Design review of the part built by this model. Coordinates are the model's own, in mm. Coordinates: 2 decimals unless noted, no trailing zeros. Order: outer loops, then holes, each group sorted by start corner. A loop starts at its lowest first (then second) coordinate and runs counter-clockwise, first axis right, second up. Notation, with made-up numbers: M 3.5,60.25 L 36.5,60.25 A26 ccw 36.5,79.25 Z; hole C 69.5,65.25 d4. An arc over 180 degrees is marked long. Answer in a Markdown table with one row per item.
from build123d import *

# Parameters (mm, degrees)
F1_DEPTH = 6.35


with BuildPart() as f1:
    # F0 (on Front) → F1 (new body)
    with BuildSketch(Plane.XZ):
        Polygon((-100.167322, -14.499216), (-100.167322, 36.300784), (-94.868163, 36.300784), (-88.733239, 36.300784), (-82.168163, 36.300784), (-76.033239, 36.300784), (-69.468163, 36.300784), (-63.333239, 36.300784), (-56.768163, 36.300784), (-50.633239, 36.300784), (-44.068163, 36.300784), (-37.933239, 36.300784), (-31.368163, 36.300784), (-25.233239, 36.300784), (-18.668163, 36.300784), (-12.533239, 36.300784), (-5.968163, 36.300784), (0.166761, 36.300784), (6.731837, 36.300784), (12.866761, 36.300784), (19.431837, 36.300784), (25.566761, 36.300784), (32.131837, 36.300784), (38.266761, 36.300784), (44.831837, 36.300784), (50.966761, 36.300784), (57.531837, 36.300784), (63.666761, 36.300784), (70.231837, 36.300784), (76.366761, 36.300784), (82.931837, 36.300784), (89.066761, 36.300784), (95.631837, 36.300784), (101.766761, 36.300784), (103.032678, 36.300784), (103.032678, 39.458872), (-106.993854, 39.458872), (-106.993854, -18.961128), (103.032678, -18.961128), (103.032678, -14.499216), (101.766761, -14.499216), (95.631837, -14.499216), (89.066761, -14.499216), (82.931837, -14.499216), (76.366761, -14.499216), (70.231837, -14.499216), (63.666761, -14.499216), (57.531837, -14.499216), (50.966761, -14.499216), (44.831837, -14.499216), (38.266761, -14.499216), (32.131837, -14.499216), (25.566761, -14.499216), (19.431837, -14.499216), (12.866761, -14.499216), (6.731837, -14.499216), (0.166761, -14.499216), (-5.968163, -14.499216), (-12.533239, -14.499216), (-18.668163, -14.499216), (-25.233239, -14.499216), (-31.368163, -14.499216), (-37.933239, -14.499216), (-44.068163, -14.499216), (-50.633239, -14.499216), (-56.768163, -14.499216), (-63.333239, -14.499216), (-69.468163, -14.499216), (-76.033239, -14.499216), (-82.168163, -14.499216), (-88.733239, -14.499216), (-94.868163, -14.499216), align=None)
        with BuildLine():
            Line((-88.733239, 36.300784), (-94.868163, 36.300784))
            ThreePointArc((-94.868163, 36.300784), (-94.016162, 33.181807), (-91.696805, 30.92914))
            ThreePointArc((-91.696805, 30.92914), (-89.523277, 33.233322), (-88.733239, 36.300784))
        make_face()
        with BuildLine():
            Line((-76.033239, 36.300784), (-82.168163, 36.300784))
            ThreePointArc((-82.168163, 36.300784), (-81.316162, 33.181807), (-78.996805, 30.92914))
            ThreePointArc((-78.996805, 30.92914), (-76.823277, 33.233322), (-76.033239, 36.300784))
        make_face()
        with BuildLine():
            Line((-63.333239, 36.300784), (-69.468163, 36.300784))
            ThreePointArc((-69.468163, 36.300784), (-68.616162, 33.181807), (-66.296805, 30.92914))
            ThreePointArc((-66.296805, 30.92914), (-64.123277, 33.233322), (-63.333239, 36.300784))
        make_face()
        with BuildLine():
            Line((-50.633239, 36.300784), (-56.768163, 36.300784))
            ThreePointArc((-56.768163, 36.300784), (-55.916162, 33.181807), (-53.596805, 30.92914))
            ThreePointArc((-53.596805, 30.92914), (-51.423277, 33.233322), (-50.633239, 36.300784))
        make_face()
        with BuildLine():
            Line((-37.933239, 36.300784), (-44.068163, 36.300784))
            ThreePointArc((-44.068163, 36.300784), (-43.216162, 33.181807), (-40.896805, 30.92914))
            ThreePointArc((-40.896805, 30.92914), (-38.723277, 33.233322), (-37.933239, 36.300784))
        make_face()
        with BuildLine():
            Line((-25.233239, 36.300784), (-31.368163, 36.300784))
            ThreePointArc((-31.368163, 36.300784), (-30.516162, 33.181807), (-28.196805, 30.92914))
            ThreePointArc((-28.196805, 30.92914), (-26.023277, 33.233322), (-25.233239, 36.300784))
        make_face()
        with BuildLine():
            Line((-12.533239, 36.300784), (-18.668163, 36.300784))
            ThreePointArc((-18.668163, 36.300784), (-17.816162, 33.181807), (-15.496805, 30.92914))
            ThreePointArc((-15.496805, 30.92914), (-13.323277, 33.233322), (-12.533239, 36.300784))
        make_face()
        with BuildLine():
            Line((0.166761, 36.300784), (-5.968163, 36.300784))
            ThreePointArc((-5.968163, 36.300784), (-5.116162, 33.181807), (-2.796805, 30.92914))
            ThreePointArc((-2.796805, 30.92914), (-0.623277, 33.233322), (0.166761, 36.300784))
        make_face()
        with BuildLine():
            Line((12.866761, 36.300784), (6.731837, 36.300784))
            ThreePointArc((6.731837, 36.300784), (7.583838, 33.181807), (9.903195, 30.92914))
            ThreePointArc((9.903195, 30.92914), (12.076723, 33.233322), (12.866761, 36.300784))
        make_face()
        with BuildLine():
            Line((25.566761, 36.300784), (19.431837, 36.300784))
            ThreePointArc((19.431837, 36.300784), (20.283838, 33.181807), (22.603195, 30.92914))
            ThreePointArc((22.603195, 30.92914), (24.776723, 33.233322), (25.566761, 36.300784))
        make_face()
        with BuildLine():
            Line((38.266761, 36.300784), (32.131837, 36.300784))
            ThreePointArc((32.131837, 36.300784), (32.983838, 33.181807), (35.303195, 30.92914))
            ThreePointArc((35.303195, 30.92914), (37.476723, 33.233322), (38.266761, 36.300784))
        make_face()
        with BuildLine():
            Line((50.966761, 36.300784), (44.831837, 36.300784))
            ThreePointArc((44.831837, 36.300784), (45.683838, 33.181807), (48.003195, 30.92914))
            ThreePointArc((48.003195, 30.92914), (50.176723, 33.233322), (50.966761, 36.300784))
        make_face()
        with BuildLine():
            Line((63.666761, 36.300784), (57.531837, 36.300784))
            ThreePointArc((57.531837, 36.300784), (58.383838, 33.181807), (60.703195, 30.92914))
            ThreePointArc((60.703195, 30.92914), (62.876723, 33.233322), (63.666761, 36.300784))
        make_face()
        with BuildLine():
            Line((76.366761, 36.300784), (70.231837, 36.300784))
            ThreePointArc((70.231837, 36.300784), (71.083838, 33.181807), (73.403195, 30.92914))
            ThreePointArc((73.403195, 30.92914), (75.576723, 33.233322), (76.366761, 36.300784))
        make_face()
        with BuildLine():
            Line((89.066761, 36.300784), (82.931837, 36.300784))
            ThreePointArc((82.931837, 36.300784), (83.783838, 33.181807), (86.103195, 30.92914))
            ThreePointArc((86.103195, 30.92914), (88.276723, 33.233322), (89.066761, 36.300784))
        make_face()
        with BuildLine():
            Line((101.766761, 36.300784), (95.631837, 36.300784))
            ThreePointArc((95.631837, 36.300784), (96.483838, 33.181807), (98.803195, 30.92914))
            ThreePointArc((98.803195, 30.92914), (100.976723, 33.233322), (101.766761, 36.300784))
        make_face()
        with BuildLine():
            ThreePointArc((98.803195, -9.127571), (96.483838, -11.380239), (95.631837, -14.499216))
            Line((95.631837, -14.499216), (101.766761, -14.499216))
            ThreePointArc((101.766761, -14.499216), (100.976723, -11.431754), (98.803195, -9.127571))
        make_face()
        with BuildLine():
            ThreePointArc((86.103195, -9.127571), (83.783838, -11.380239), (82.931837, -14.499216))
            Line((82.931837, -14.499216), (89.066761, -14.499216))
            ThreePointArc((89.066761, -14.499216), (88.276723, -11.431754), (86.103195, -9.127571))
        make_face()
        with BuildLine():
            ThreePointArc((73.403195, -9.127571), (71.083838, -11.380239), (70.231837, -14.499216))
            Line((70.231837, -14.499216), (76.366761, -14.499216))
            ThreePointArc((76.366761, -14.499216), (75.576723, -11.431754), (73.403195, -9.127571))
        make_face()
        with BuildLine():
            ThreePointArc((60.703195, -9.127571), (58.383838, -11.380239), (57.531837, -14.499216))
            Line((57.531837, -14.499216), (63.666761, -14.499216))
            ThreePointArc((63.666761, -14.499216), (62.876723, -11.431754), (60.703195, -9.127571))
        make_face()
        with BuildLine():
            ThreePointArc((48.003195, -9.127571), (45.683838, -11.380239), (44.831837, -14.499216))
            Line((44.831837, -14.499216), (50.966761, -14.499216))
            ThreePointArc((50.966761, -14.499216), (50.176723, -11.431754), (48.003195, -9.127571))
        make_face()
        with BuildLine():
            ThreePointArc((35.303195, -9.127571), (32.983838, -11.380239), (32.131837, -14.499216))
            Line((32.131837, -14.499216), (38.266761, -14.499216))
            ThreePointArc((38.266761, -14.499216), (37.476723, -11.431754), (35.303195, -9.127571))
        make_face()
        with BuildLine():
            ThreePointArc((22.603195, -9.127571), (20.283838, -11.380239), (19.431837, -14.499216))
            Line((19.431837, -14.499216), (25.566761, -14.499216))
            ThreePointArc((25.566761, -14.499216), (24.776723, -11.431754), (22.603195, -9.127571))
        make_face()
        with BuildLine():
            ThreePointArc((9.903195, -9.127571), (7.583838, -11.380239), (6.731837, -14.499216))
            Line((6.731837, -14.499216), (12.866761, -14.499216))
            ThreePointArc((12.866761, -14.499216), (12.076723, -11.431754), (9.903195, -9.127571))
        make_face()
        with BuildLine():
            ThreePointArc((-2.796805, -9.127571), (-5.116162, -11.380239), (-5.968163, -14.499216))
            Line((-5.968163, -14.499216), (0.166761, -14.499216))
            ThreePointArc((0.166761, -14.499216), (-0.623277, -11.431754), (-2.796805, -9.127571))
        make_face()
        with BuildLine():
            ThreePointArc((-15.496805, -9.127571), (-17.816162, -11.380239), (-18.668163, -14.499216))
            Line((-18.668163, -14.499216), (-12.533239, -14.499216))
            ThreePointArc((-12.533239, -14.499216), (-13.323277, -11.431754), (-15.496805, -9.127571))
        make_face()
        with BuildLine():
            ThreePointArc((-28.196805, -9.127571), (-30.516162, -11.380239), (-31.368163, -14.499216))
            Line((-31.368163, -14.499216), (-25.233239, -14.499216))
            ThreePointArc((-25.233239, -14.499216), (-26.023277, -11.431754), (-28.196805, -9.127571))
        make_face()
        with BuildLine():
            ThreePointArc((-40.896805, -9.127571), (-43.216162, -11.380239), (-44.068163, -14.499216))
            Line((-44.068163, -14.499216), (-37.933239, -14.499216))
            ThreePointArc((-37.933239, -14.499216), (-38.723277, -11.431754), (-40.896805, -9.127571))
        make_face()
        with BuildLine():
            ThreePointArc((-53.596805, -9.127571), (-55.916162, -11.380239), (-56.768163, -14.499216))
            Line((-56.768163, -14.499216), (-50.633239, -14.499216))
            ThreePointArc((-50.633239, -14.499216), (-51.423277, -11.431754), (-53.596805, -9.127571))
        make_face()
        with BuildLine():
            ThreePointArc((-66.296805, -9.127571), (-68.616162, -11.380239), (-69.468163, -14.499216))
            Line((-69.468163, -14.499216), (-63.333239, -14.499216))
            ThreePointArc((-63.333239, -14.499216), (-64.123277, -11.431754), (-66.296805, -9.127571))
        make_face()
        with BuildLine():
            ThreePointArc((-78.996805, -9.127571), (-81.316162, -11.380239), (-82.168163, -14.499216))
            Line((-82.168163, -14.499216), (-76.033239, -14.499216))
            ThreePointArc((-76.033239, -14.499216), (-76.823277, -11.431754), (-78.996805, -9.127571))
        make_face()
        with BuildLine():
            ThreePointArc((-91.696805, -9.127571), (-94.016162, -11.380239), (-94.868163, -14.499216))
            Line((-94.868163, -14.499216), (-88.733239, -14.499216))
            ThreePointArc((-88.733239, -14.499216), (-89.523277, -11.431754), (-91.696805, -9.127571))
        make_face()
    extrude(amount=F1_DEPTH)


solid = f1.part
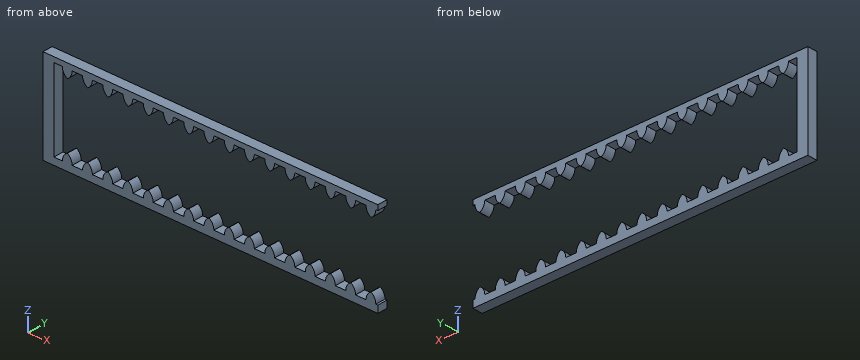
(1) Add section B-B, the plane z = 18. Give the boundary of the cut face in (x, y).
Return value:
| item | result |
|---|---|
| outline | M -106.99,-6.35 L -100.17,-6.35 L -100.17,0 L -106.99,0 Z |
(2) For line 1 along Z through (x, y) = (-7.5, -2.25); line 2 along X through (y, z) = (-5, -4); line 3 along Z through (x, y) = (74, -2.5), list the stretches that pass through material, from the lowest coordinate up. Write a range as from..to.
Return value:
| item | result |
|---|---|
| line 1 | z = -18.96..-14.5, 36.3..39.46 |
| line 2 | x = -106.99..-100.17 |
| line 3 | z = -18.96..-9.55, 31.36..39.46 |
(3) Add section A-A, the plane x = 67. Give the boundary of the cut face in (y, z).
Return value:
| item | result |
|---|---|
| outline | M -6.35,-18.96 L 0,-18.96 L 0,-14.5 L -6.35,-14.5 Z; M -6.35,36.3 L 0,36.3 L 0,39.46 L -6.35,39.46 Z |
